Drawing for the job (mm, zero at the part's lowest x, y, z). A direction names the side the tool comes from. Round coordinates to 2 decimals unless told otherwise and drop trailing zeros. Write each loop counter-clockwise with the first axis right and the second up, starting at its lowest first coordinate (ties: lowest second). Pieces come first, ordered by that corner, then holes. Notation, with made-up numbers: (-18.75, 88) - (26.25, 88) arc R12 ccw to (26.25, 107) - close; hole circle Ø4 at (3, 8). An arc over 180 degrees is marked (long way). One line per question, with ' | ' between items.
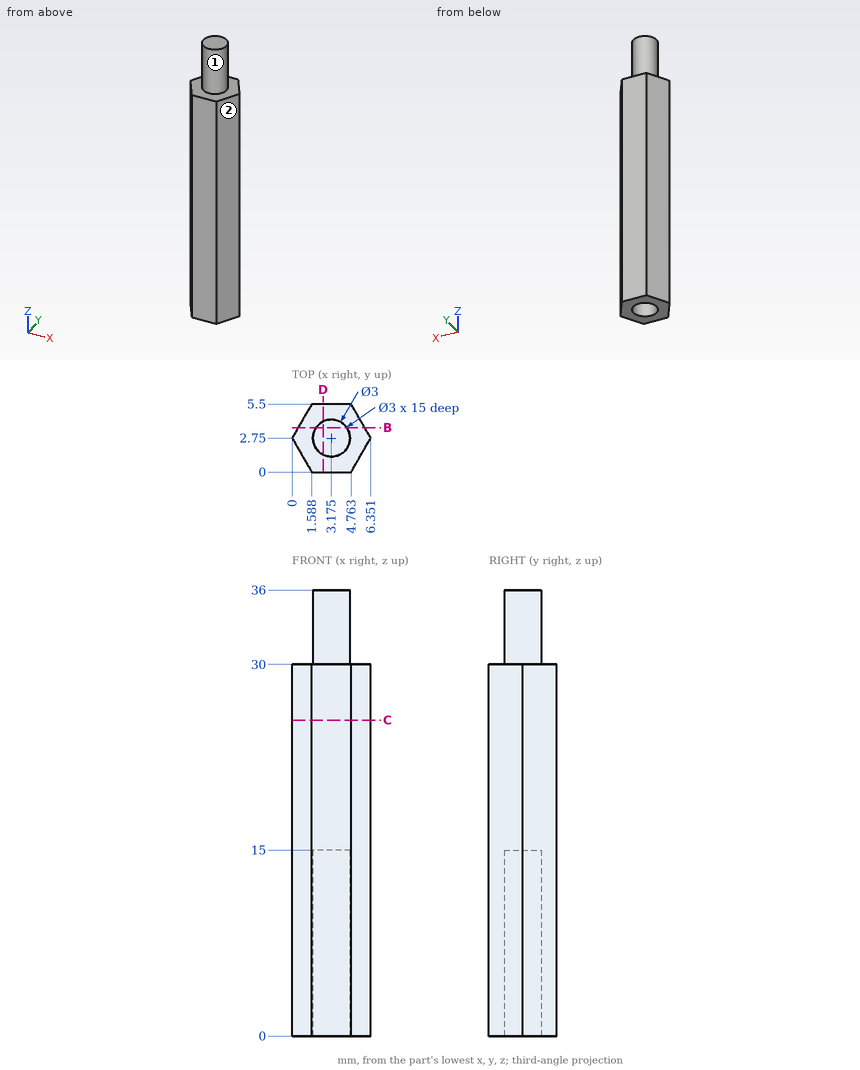
Q1. Drill centre lines: L1, parallel to Z at x = 2, y = 3.25; L2, parallel to Z at x = 4.5, y = 1; L3, parallel to Y at x = 1, z = 13 (1 decimal). Where is each one in solid material? Low to high. Write a range as from..to.
Found:
L1: 15..36 | L2: 0..30 | L3: 1..4.5
Q2. Saw through at D-D, the plane x = 2.5. List the corners of the cut face in (y, z), then the cut area to 3 significant figures.
Found:
outline: (0, 0) - (1.41, 0) - (1.41, 15) - (4.09, 15) - (4.09, 0) - (5.5, 0) - (5.5, 30) - (4.09, 30) - (4.09, 36) - (1.41, 36) - (1.41, 30) - (0, 30) - close | area: 141 mm^2
Q3. Drop flat-ended pins along their axis: pin 1 (3 mm diameter, centred on y = 1, z = 4, fed in from +X); pin 2 (2 mm diameter, centred on y = 4.5, z = 30.5, fed in from -X); pin 3 (1.5 mm diameter, centred on y = 1, z = 7.5, fed in from +X). Give the stop position or say it passes through.
Found:
pin 1: x = 6.21 | pin 2: x = 0.51 | pin 3: x = 5.77
Q4. Which spindle directions (+Z, -Z, +X, -X, +Y, -Y) get a long thin tool onto all of the face, cutting with end or side? Do the marked faces 1 and 2. Say none if no direction does.
Found:
face 1: +Z | face 2: +Z, -Z, +X, -Y
Q5. Saw through at B-B, the plane y = 3.6. List the corners of the cut face in (x, z).
Found:
outline: (0.49, 0) - (1.94, 0) - (1.94, 15) - (4.41, 15) - (4.41, 0) - (5.86, 0) - (5.86, 30) - (4.41, 30) - (4.41, 36) - (1.94, 36) - (1.94, 30) - (0.49, 30) - close
Q6. Saw through at C-C, the plane z = 25.5. List the corners of the cut face in (x, y), then the cut area to 3 significant figures.
Found:
outline: (0, 2.75) - (1.59, 0) - (4.76, 0) - (6.35, 2.75) - (4.76, 5.5) - (1.59, 5.5) - close | area: 26.2 mm^2
